The model under review builds one solid part; all positions refer to its coordinate system, in mm. A direction names the side the tool comes from. Coordinates: 2 decimals unless noted, no trailing zeros. Write each loop counter-clockwise with the first axis right and the second up, starting at its lowest first coordinate (ties: lowest second). Pieces come first, ordered by that corner, then holes.
1) For P1, Ø0.6, axis at y = 15.5, z = 1, coming from the -X side; P2, Ø0.6, axis at x = -22.5, z = 1, coming from the -Y side; P3, Ø1, axis at x = -46.5, z = 1.5, coming from the +Y side, all flat-tipped, find the tip position at first contact; note any pin that passes through.
2) Mouldability with a two-part tool opening along Y and no side actions: class faces 1 (the flat face through (49, -0.143, 1)), 2 (the cylindrical face through (21.5, 18.5, 1)), 3 (the flat face through (-1, 19, 0)), 4 (the flat face through (-30, 34.6, 1)) as released by +Y, released by -Y, zero draft, split by the parting line, or undercut.
3) Add section C-C, the plane y = 28.5. State the section outline as (x, z) points.
4) For line 1 (X direction, y = 16, z = 1.1); line 2 (Y direction, x = 8, z = 0.7); line 3 (X direction, y = 9, z = 1.1), list the stretches that pass through material, from the lowest coordinate up.
5) Add section D-D, the plane x = 21.5. State the section outline as (y, z) points.
6) Add section A-A, the plane y = 3. State the section outline as (x, z) points, then the cut area to 3 significant figures.
7) Machinability: for faces 5 (the flat face through (-22, 15, 1)), 6 (the flat face through (13, 32, 1)), 7 (the flat face through (26.7, 2.46, 0.99)), which of the approach directions +Z, -Z, +X, -X, +Y, -Y give a long, thin tool a straight path to every point of the face, cutting with its end or side? Answer none if there is none.
8) Add section B-B, the plane x = -39.5. State the section outline as (y, z) points, then the cut area to 3 significant figures.
from build123d import *

# Parameters (mm, degrees)
RESSALTO_EXTRUS_O1_DEPTH = 2
ESBO_O2_R                = 1.5
ESBO_O2_W                = 22
ESBO_O2_H                = 2
CORTE_EXTRUS_O1_DEPTH    = 3


with BuildPart() as part:
    # Esboço1 → Ressalto-extrusão1 (new body)
    with BuildSketch(Plane.XY):
        with BuildLine():
            Line((52, -0.143401487), (45, -0.143401487))
            Line((45, -0.143401487), (41, 4.856598513))
            Line((41, 4.856598513), (12, 0))
            Line((12, 0), (0, 0))
            Line((0, 0), (0, 27))
            Line((0, 27), (9, 27))
            Line((9, 27), (17, 37))
            Line((17, 37), (27, 37))
            Line((27, 37), (33, 32.2))
            Line((33, 32.2), (60, 23.856598513))
            Line((60, 23.856598513), (60, 7.856598513))
            ThreePointArc((60, 7.856598513), (57.656854249, 2.199744264), (52, -0.143401487))
        make_face()
    ressalto_extrus_o1 = extrude(amount=RESSALTO_EXTRUS_O1_DEPTH)

    # Espelhar1: Ressalto-extrusão1 across plane
    add(ressalto_extrus_o1.mirror(Plane(origin=(0, 0, 0), x_dir=(0, 0, 1), z_dir=(1, 0, 0))))

    # Esboço2 → Corte-extrusão1 (cut, through all)
    with BuildSketch(Plane.XY.offset(2)):
        with Locations((8, 8)):
            Circle(ESBO_O2_R)
        with Locations((-8, 8)):
            Circle(ESBO_O2_R)
        with Locations((49, 15.856598513)):
            Rectangle(ESBO_O2_W, ESBO_O2_H)
        with BuildLine():
            Line((23, 35), (23, 20))
            ThreePointArc((23, 20), (21.5, 18.5), (20, 20))
            Line((20, 20), (20, 35))
            ThreePointArc((20, 35), (21.5, 36.5), (23, 35))
        make_face()
        with BuildLine():
            Line((25, 15), (18, 15))
            ThreePointArc((18, 15), (17, 16), (18, 17))
            Line((18, 17), (25, 17))
            ThreePointArc((25, 17), (26, 16), (25, 15))
        make_face()
        with BuildLine():
            Line((-23, 35), (-23, 20))
            ThreePointArc((-23, 20), (-21.5, 18.5), (-20, 20))
            Line((-20, 20), (-20, 35))
            ThreePointArc((-20, 35), (-21.5, 36.5), (-23, 35))
        make_face()
        with BuildLine():
            Line((-25, 15), (-18, 15))
            ThreePointArc((-18, 15), (-17, 16), (-18, 17))
            Line((-18, 17), (-25, 17))
            ThreePointArc((-25, 17), (-26, 16), (-25, 15))
        make_face()
        with Locations((-49, 15.856598513)):
            Rectangle(ESBO_O2_W, ESBO_O2_H)
    extrude(amount=-CORTE_EXTRUS_O1_DEPTH, mode=Mode.SUBTRACT)


solid = part.part
Geometry results:
1. P1: stops at x = -38
1. P2: stops at y = 1.71
1. P3: stops at y = 28.18
2. face 1: released by -Y
2. face 2: undercut
2. face 3: zero draft
2. face 4: released by +Y
3. outline: (-44.97, 0) - (-23, 0) - (-23, 2) - (-44.97, 2) - close; (-20, 0) - (-10.2, 0) - (-10.2, 2) - (-20, 2) - close; (10.2, 0) - (20, 0) - (20, 2) - (10.2, 2) - close; (23, 0) - (44.97, 0) - (44.97, 2) - (23, 2) - close
4. line 1: x = -38 to -26, -17 to 17, 26 to 38
4. line 2: y = 0 to 6.5, 9.5 to 27
4. line 3: x = -60 to -9.12, -6.88 to 6.88, 9.12 to 60
5. outline: (1.59, 0) - (15, 0) - (15, 2) - (1.59, 2) - close; (17, 0) - (18.5, 0) - (18.5, 2) - (17, 2) - close; (36.5, 0) - (37, 0) - (37, 2) - (36.5, 2) - close
6. outline: (-58.36, 0) - (-42.49, 0) - (-42.49, 2) - (-58.36, 2) - close; (-29.91, 0) - (29.91, 0) - (29.91, 2) - (-29.91, 2) - close; (42.49, 0) - (58.36, 0) - (58.36, 2) - (42.49, 2) - close
6. area: 183 mm2
7. face 5: +Z, -Z
7. face 6: +Z, -Z, +Y
7. face 7: +Z, -Z, -Y
8. outline: (4.61, 0) - (14.86, 0) - (14.86, 2) - (4.61, 2) - close; (16.86, 0) - (30.19, 0) - (30.19, 2) - (16.86, 2) - close
8. area: 47.2 mm2
